from build123d import *

# Parameters (mm, degrees)
SKETCH_1_W           = 20
SKETCH_1_H           = 20
EXTRUDE_1_DEPTH      = 4
SKETCH_2_W           = 12.9
SKETCH_2_H           = 20
EXTRUDE_2_DEPTH      = 4.5
SKETCH_3_R           = 1.6
CUT_EXTRUDE_1_DEPTH  = 30.533878851
SKETCH_4_W           = 5.8
SKETCH_4_H           = 20
SKETCH_4_R           = 1.6
EXTRUDE_3_DEPTH      = 2
SKETCH_5_R           = 3
CUT_EXTRUDE_3_DEPTH  = 2.4
SKETCH_6_W           = 20
SKETCH_6_H           = 4
EXTRUDE_4_DEPTH      = 3
EXTRUDE_START        = 4
SKETCH_7_W           = 23
SKETCH_7_H           = 20
SKETCH_7_R           = 3
EXTRUDE_5_DEPTH      = 4
SKETCH_9_W           = 10.1
SKETCH_9_H           = 20
EXTRUDE_6_DEPTH      = 2
EXTRUDE_7_DEPTH      = 5
CHAMFER_7_SIZE       = 10
CHAMFER_7_SIZE2      = 5.773502692
CHAMFER_8_SIZE       = 5
CHAMFER_9_SIZE       = 8
CHAMFER_9_SIZE2      = 4.618802154
CUT_EXTRUDE_9_DEPTH  = 10.1
CUT_EXTRUDE_10_REACH = 38.936
CHAMFER_10_SIZE      = 1.5


with BuildPart() as part:
    # 草图1 → 凸台-拉伸1 (new body)
    with BuildSketch(Plane(origin=(0, 0, 0), x_dir=(1, 0, 0), z_dir=(0, 1, 0))):
        with Locations((10, 10)):
            Rectangle(SKETCH_1_W, SKETCH_1_H)
    extrude(amount=EXTRUDE_1_DEPTH)

    # 草图2 → 凸台-拉伸2 (add)
    with BuildSketch(Plane(origin=(0, 4, 0), x_dir=(1, 0, 0), z_dir=(0, 1, 0))):
        with Locations((6.45, 10)):
            Rectangle(SKETCH_2_W, SKETCH_2_H)
    extrude(amount=EXTRUDE_2_DEPTH)

    # 草图3 → 切除-拉伸1 (cut, through all)
    with BuildSketch(Plane(origin=(0, 0, 0), x_dir=(-1, 0, 0), z_dir=(0, -1, 0))):
        with Locations(Location((-10, 5, 0), (0, 0, 90))):
            Circle(SKETCH_3_R)
        with Locations(Location((-10, 13, 0), (0, 0, 90))):
            Circle(SKETCH_3_R)
    extrude(amount=-CUT_EXTRUDE_1_DEPTH, mode=Mode.SUBTRACT)

    # 草图4 → 凸台-拉伸3 (add)
    with BuildSketch(Plane(origin=(0, 8.5, 0), x_dir=(1, 0, 0), z_dir=(0, 1, 0))):
        with Locations((10, 10)):
            Rectangle(SKETCH_4_W, SKETCH_4_H)
        with Locations(Location((10, 13, 0), (0, 0, 90))):
            Circle(SKETCH_4_R, mode=Mode.SUBTRACT)
        with Locations(Location((10, 5, 0), (0, 0, 90))):
            Circle(SKETCH_4_R, mode=Mode.SUBTRACT)
    extrude(amount=EXTRUDE_3_DEPTH)

    # 草图5 → 切除-拉伸3 (cut)
    with BuildSketch(Plane(origin=(0, 0, 0), x_dir=(-1, 0, 0), z_dir=(0, -1, 0))):
        with Locations(Location((-10, 5, 0), (0, 0, 90))):
            Circle(SKETCH_5_R)
        with Locations(Location((-10, 13, 0), (0, 0, 90))):
            Circle(SKETCH_5_R)
    extrude(amount=-CUT_EXTRUDE_3_DEPTH, mode=Mode.SUBTRACT)

    # 草图6 → 凸台-拉伸4 (add)
    with BuildSketch(Plane(origin=(20, 0, 0), x_dir=(0, 0, -1), z_dir=(1, 0, 0))):
        with Locations((10, 2)):
            Rectangle(SKETCH_6_W, SKETCH_6_H)
    extrude(amount=EXTRUDE_4_DEPTH)

    # 草图7 → 凸台-拉伸5 (add)
    with BuildSketch(Plane(origin=(0, 0, 0), x_dir=(-1, 0, 0), z_dir=(0, -1, 0)).offset(EXTRUDE_START)):
        with Locations((-11.5, 10)):
            Rectangle(SKETCH_7_W, SKETCH_7_H)
        with Locations(Location((-10, 13, 0), (0, 0, 90))):
            Circle(SKETCH_7_R, mode=Mode.SUBTRACT)
        with Locations(Location((-10, 5, 0), (0, 0, 90))):
            Circle(SKETCH_7_R, mode=Mode.SUBTRACT)
    extrude(amount=-EXTRUDE_5_DEPTH)

    # 草图9 → 凸台-拉伸6 (add)
    with BuildSketch(Plane(origin=(0, 4, 0), x_dir=(1, 0, 0), z_dir=(0, 1, 0))):
        with Locations((17.95, 10)):
            Rectangle(SKETCH_9_W, SKETCH_9_H)
    extrude(amount=EXTRUDE_6_DEPTH)

    # 草图11 → 凸台-拉伸7 (add)
    with BuildSketch(Plane(origin=(0, 0, -20), x_dir=(-1, 0, 0), z_dir=(0, 0, -1))):
        Polygon((-23, 6), (-23, -4), (0, -4), (0, 8.5), (-7.1, 8.5), (-7.1, 10.5), (-12.9, 10.5), (-12.9, 6), align=None)
    extrude(amount=EXTRUDE_7_DEPTH)

    # 倒角7
    chamfer_7_edges = [part.edges().sort_by_distance(p)[0] for p in [
        (0, -4, -12.5),
    ]]
    chamfer_7_side = [part.faces().sort_by_distance(p)[0] for p in [
        (0, 2.25, -12.5),
    ]]
    chamfer(chamfer_7_edges, length=CHAMFER_7_SIZE, length2=CHAMFER_7_SIZE2, reference=chamfer_7_side[0])

    # 倒角8
    chamfer_8_edges = [part.edges().sort_by_distance(p)[0] for p in [
        (23, 1, 0),
    ]]
    chamfer(chamfer_8_edges, length=CHAMFER_8_SIZE)

    # 倒角9
    chamfer_9_edges = [part.edges().sort_by_distance(p)[0] for p in [
        (20.5, -4, -2.5),
    ]]
    chamfer_9_side = [part.faces().sort_by_distance(p)[0] for p in [
        (20.5, 1, -2.5),
    ]]
    chamfer(chamfer_9_edges, length=CHAMFER_9_SIZE, length2=CHAMFER_9_SIZE2, reference=chamfer_9_side[0])

    # 草图15 → 切除-拉伸9 (cut)
    with BuildSketch(Plane(origin=(23, 0, 0), x_dir=(0, 0, -1), z_dir=(1, 0, 0))):
        Polygon((25, -3), (25, 6), (7, 6), align=None)
    extrude(amount=-CUT_EXTRUDE_9_DEPTH, mode=Mode.SUBTRACT)

    # 切除-拉伸10: up to this plane
    cut_extrude_10_end = Plane(origin=(-7.224611797, 6, -7), z_dir=(0, -0.894427190999916, 0.447213595499958))
    # 草图16 → 切除-拉伸10 (cut, up to the surface)
    with BuildSketch(Plane(origin=(0, 10.5, 0), x_dir=(1, 0, 0), z_dir=(0, 1, 0)), mode=Mode.PRIVATE) as cut_extrude_10_sk1:
        Polygon((7.9, 25), (12.9, 25), (12.9, 14), align=None)
    cut_extrude_10_tool1 = split(extrude(cut_extrude_10_sk1.sketch, amount=-CUT_EXTRUDE_10_REACH, mode=Mode.PRIVATE), bisect_by=cut_extrude_10_end, keep=Keep.BOTH, mode=Mode.PRIVATE)
    add(cut_extrude_10_tool1.solids().sort_by_distance((11.233333, 10.5, -21.333333))[0], mode=Mode.SUBTRACT)

    # 倒角10
    # the kernel refuses this chamfer: 1.5 mm, written as the material it takes off along each edge
    with BuildSketch(Plane(origin=(10, 2.4, -13), x_dir=(0, 0, -1), z_dir=(-1, 0, 0))) as chamfer_10_piece_1_section:
        Polygon((1.6, -CHAMFER_10_SIZE), (1.6 + CHAMFER_10_SIZE, 0), (1.6, 0), align=None)
    chamfer_10_piece_1 = revolve(axis=Axis((10, 2.4, -13), (0, -1, 0)), mode=Mode.PRIVATE)
    chamfer_10_piece_1 = chamfer_10_piece_1 & Plane(origin=(10, 3.20338318, -13), x_dir=(0, 0, -1), z_dir=(0, -1, 0)) * Cylinder(3, 13, mode=Mode.PRIVATE)
    add(chamfer_10_piece_1, mode=Mode.SUBTRACT)
    with BuildSketch(Plane(origin=(10, 2.4, -5), x_dir=(0, 0, -1), z_dir=(-1, 0, 0))) as chamfer_10_piece_2_section:
        Polygon((1.6, -CHAMFER_10_SIZE), (1.6 + CHAMFER_10_SIZE, 0), (1.6, 0), align=None)
    chamfer_10_piece_2 = revolve(axis=Axis((10, 2.4, -5), (0, -1, 0)), mode=Mode.PRIVATE)
    chamfer_10_piece_2 = chamfer_10_piece_2 & Plane(origin=(10, 3.20338318, -5), x_dir=(0, 0, -1), z_dir=(0, -1, 0)) * Cylinder(3, 13, mode=Mode.PRIVATE)
    add(chamfer_10_piece_2, mode=Mode.SUBTRACT)


solid = part.part
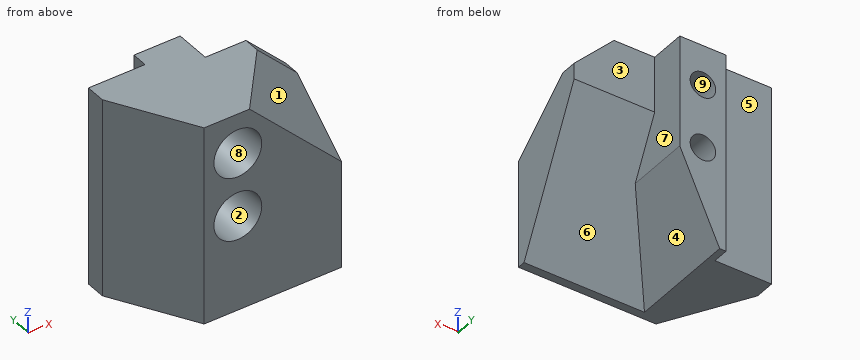
The model under review builds one solid part; all positions refer to its coordinate system, in mm. Face numbers are marked on the shaded views. A direction names the side the tool comes from. Give positions to 0.01 mm unless a question says otherwise; leave off trailing zeros. Loops run counter-clockwise (first coordinate to the right, second up) from the corner with the lowest first, then second, coordinate; pieces in that order, holes last. Notation, with made-up numbers: (-18, -36.5) -> (26, -36.5) arc R12 ccw to (26, -28.5) -> close; hole circle Ø10 at (2.5, 14.25). An arc over 180 degrees is marked (long way). Write each question's results on one line, items separated by ' | '.
1) Tool access review of the marked faces 1, 2, 3, 4 and 5: name each direction out of +Z, -Z, +X, -X, +Y, -Y from which nothing blocks a thin tool from reaching the whole face with its end or side.
Conclusion:
face 1: +Z, +X, -Y | face 2: -Y | face 3: +Z, -Z, +X, +Y | face 4: -Z, +X, +Y | face 5: +Z, -Z, -X, +Y
2) Take a section at A-A, the plane y = 7.5. Give the boundary of the cut face in (x, z), plus the area to 3 significant figures.
Conclusion:
outline: (0, -25) -> (7.9, -25) -> (12.9, -14) -> (12.9, 0) -> (0, 0) -> close; hole circle Ø3.2 at (10, -13); hole circle Ø3.2 at (10, -5) | area: 279 mm^2
3) Take a section at D-D, the plane y = 9. Give the boundary of the cut face in (x, z).
Conclusion:
outline: (7.1, -25) -> (7.9, -25) -> (12.9, -14) -> (12.9, 0) -> (7.1, 0) -> close; hole circle Ø3.2 at (10, -13); hole circle Ø3.2 at (10, -5)
4) Draft analysis for pull direction X (two halves, no side actions). For the marked faces 6, 7, 8 and 9, state which applies: pulls with the +X half, pulls with the -X half, needs draft (parallel to the pull), parting line crosses it, or undercut.
Conclusion:
face 6: needs draft | face 7: pulls with the +X half | face 8: undercut | face 9: undercut
5) Take a section at B-B, the plane z = -13. Give the boundary of the cut face in (x, y).
Conclusion:
outline: (0, 6) -> (5.77, -4) -> (7, -4) -> (7, 2.5) -> (8.4, 3.9) -> (8.4, 10.5) -> (7.1, 10.5) -> (7.1, 8.5) -> (0, 8.5) -> close; (11.6, 3.9) -> (13, 2.5) -> (13, -4) -> (23, -4) -> (23, 3) -> (12.9, 3) -> (12.9, 10.5) -> (11.6, 10.5) -> close
6) Insertion check: pin 1 Ø7.5 at (x, z) = (19, -3) entering from +Y; pin 2 Ø1 at (x, y) = (17.5, -2.5) entering from +Z; pin 3 Ø1 at (x, y) = (14, 8.5) entering from +Z; pin 4 Ø1.5 at (x, z) = (18, -14) entering from +Y (3 decimals). Each pin has a flat end and moves straight along its axis. Give the tip position at first contact, or say it passes through.
Conclusion:
pin 1: stops at y = 6 | pin 2: stops at z = -4.16 | pin 3: passes through | pin 4: stops at y = 2.875
7) For line 1 along X through (y, z) = (7.5, -5); line 2 along Z through (x, y) = (10, 6.75); line 3 along X through (y, z) = (9, -13), list the stretches that pass through material, from the lowest coordinate up. Write a range as from..to.
Conclusion:
line 1: x = 0..8.4, 11.6..12.9 | line 2: z = -20.38..-14.6, -11.4..-6.6, -3.4..0 | line 3: x = 7.1..8.4, 11.6..12.9
8) Take a section at C-C, the plane x = 10. Give the boundary of the cut face in (y, z), plus the area to 3 significant figures.
Conclusion:
outline: (-4, -25) -> (-3, -25) -> (-0.69, -20.38) -> (10.5, -20.38) -> (10.5, -14.6) -> (3.9, -14.6) -> (2.5, -16) -> (-4, -16) -> close; (-4, -10) -> (2.5, -10) -> (3.9, -11.4) -> (10.5, -11.4) -> (10.5, -6.6) -> (3.9, -6.6) -> (2.5, -8) -> (-4, -8) -> close; (-4, -2) -> (2.5, -2) -> (3.9, -3.4) -> (10.5, -3.4) -> (10.5, 0) -> (-4, 0) -> close | area: 172 mm^2
